Design review of the part built by this model. Coordinates are the model's own, in mm. Face numbers are marked on the shaded views. A direction names the side the tool comes from. Give positions to 0.01 mm unless a question says otherwise; leave off trailing zeros. Write each loop counter-clockwise with the first axis right and the second up, starting at its lowest first coordinate (ties: lowest second). Pieces come first, ordered by that corner, then holes. Notation, with made-up numbers: (-5.75, 83) -> (24.25, 83) arc R34 cw to (24.25, 118) -> close; hole circle Ø6 at (11.25, -17). An arc over 180 degrees is marked (long way). Answer as a JSON object with one key per item and string values.
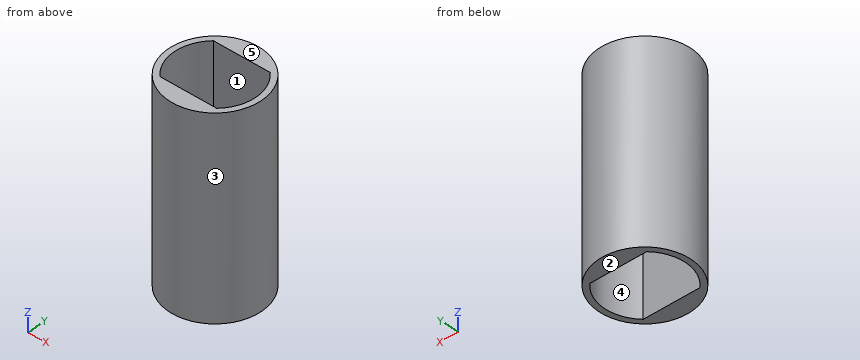
Autodesk Fusion 360 part; units mm, degrees
sketch "Spacer_Wheel_Ax_Sketch" plane through (0, 0, 0) normal (0, 0, 1) x (1, 0, 0)
  circle A0 centre (0, 0) radius 5
  arc A1 (-3, 3) -> (-3, -3) centre (0, 0) ccw
  line L0 (3, 3) -> (-3, 3)
  arc A2 (3, -3) -> (3, 3) centre (0, 0) ccw
  line L1 (-3, -3) -> (3, -3)
  line L2 (-3.0615, -3.15) -> (3.0615, -3.15)
  arc A3 (3.0615, -3.15) -> (3.0615, 3.15) centre (0, 0) ccw
  line L3 (3.0615, 3.15) -> (-3.0615, 3.15)
  arc A4 (-3.0615, 3.15) -> (-3.0615, -3.15) centre (0, 0) ccw
  dimension "d1" = 0.15
extrude "Extrude1" add sketch "Spacer_Wheel_Ax_Sketch" along normal blind 21.2 contours A0
(1) For the marked faces 1 and 2, list the 3-axis set-ups (+Z, -Z, +X, -X, +Y, -Y) from which the entire face can be reached by the end or side of a thin tool; tool diameter is ignored.
Here are the results:
{"face 1": "+Z, -Z", "face 2": "-Z, +X, -X, +Y, -Y"}
(2) We need section A-A, the plane x = 0. State the section outline as (y, z) points, then the cut area to 3 significant figures.
Here are the results:
{"outline": "(-5, 0) -> (-3.15, 0) -> (-3.15, 21.2) -> (-5, 21.2) -> close; (3.15, 0) -> (5, 0) -> (5, 21.2) -> (3.15, 21.2) -> close", "area": "78.4 mm²"}
(3) We need section C-C, the plane z = 1.5. State the section outline as (x, y) points.
Here are the results:
{"outline": "circle Ø10 at (0, 0); hole (-3.06, -3.15) -> (3.06, -3.15) arc R4.39 ccw to (3.06, 3.15) -> (-3.06, 3.15) arc R4.39 ccw to start"}
(4) We need section B-B, the plane y = -1. State the section outline as (x, z) points.
Here are the results:
{"outline": "(-4.9, 0) -> (-4.28, 0) -> (-4.28, 21.2) -> (-4.9, 21.2) -> close; (4.28, 0) -> (4.9, 0) -> (4.9, 21.2) -> (4.28, 21.2) -> close"}
(5) The part is to be moulded in two halves that separate along Y. For the marked faces 3, 4 and 5, say which applies: +Y half, -Y half, draft (parallel to the pull), parting line (faces both ways), or undercut.
Here are the results:
{"face 3": "parting line", "face 4": "undercut", "face 5": "draft"}
(6) Clearance check with flat-ended pins moving along their axes: pin 1 (2 mm diameter, centred on y = -2.5, z = 18.5, fed in from +X); pin 2 (1 mm diameter, centred on x = -3.5, y = -1.5, fed in from +Z); pin 3 (5 mm diameter, centred on x = 4, z = 13.5, fed in from +Y). State where each tip first meets the part, or that it passes through.
Here are the results:
{"pin 1": "stops at x = 4.77", "pin 2": "passes through", "pin 3": "stops at y = 4.77"}
(7) For line 1 along X through (y, z) = (3, 19.75); line 2 along Y through (x, z) = (-1, 18.25); line 3 along X through (y, z) = (-1, 13.5), list the stretches that pass through material, from the lowest coordinate up.
Here are the results:
{"line 1": "x = -4 to -3.21, 3.21 to 4", "line 2": "y = -4.9 to -3.15, 3.15 to 4.9", "line 3": "x = -4.9 to -4.28, 4.28 to 4.9"}
